For this review, use the dimensioned drawing (mm, ordinates from the lowest corner) and the shaded views. A direction names the side the tool comes from. Round coordinates to 2 decimals unless told otherwise and drop trailing zeros. Loops run counter-clockwise (first coordinate to the right, second up) from the corner with the lowest first, then second, coordinate; pieces in that order, holes last. Notation, with made-up numbers: (46, 50.5) - (100, 50.5) arc R29 ccw to (100, 70.5) - close; hole circle Ø2 at (55, 39). An arc over 180 degrees is marked (long way). Use one line per item in the form item = value. Start each with the question number.
(1) We need section C-C, the plane y = 14. Write out the cut boundary in (x, z).
(2) We need section B-B, the plane z = 21. Write out the cut boundary in (x, y) (1 decimal), then the cut area to 3 significant figures.
(3) We need section A-A, the plane x = 21. Write out the cut boundary in (y, z) (1 decimal), then the cut area to 3 significant figures.
(4) Machinability: for the marked faces 1 and 2, which of the approach directions +Z, -Z, +X, -X, +Y, -Y give a long, thin tool a straight path to every point of the face, cutting with its end or side? Answer none if there is none.
(5) For pin 1 (1.5 mm diameter, centred on x = 39.5, z = 43, fed in from -Y), flat-tipped, find the tip position at first contact; note if it passes through.
(6) Wall thickness on probe 1 along Y at (x, z) = (55, 10); probe 2 along Z at (x, y) = (30, 14.5) (1 decimal); probe 3 along Z at (x, y) = (21.5, 3.5) (1 decimal): over which ranges is each line inside the solid? List them lowest first. Write a range as [from, to].
(7) We need section D-D, the plane x = 12.5. Write out the cut boundary in (y, z) (1 decimal), then the cut area to 3 significant figures.
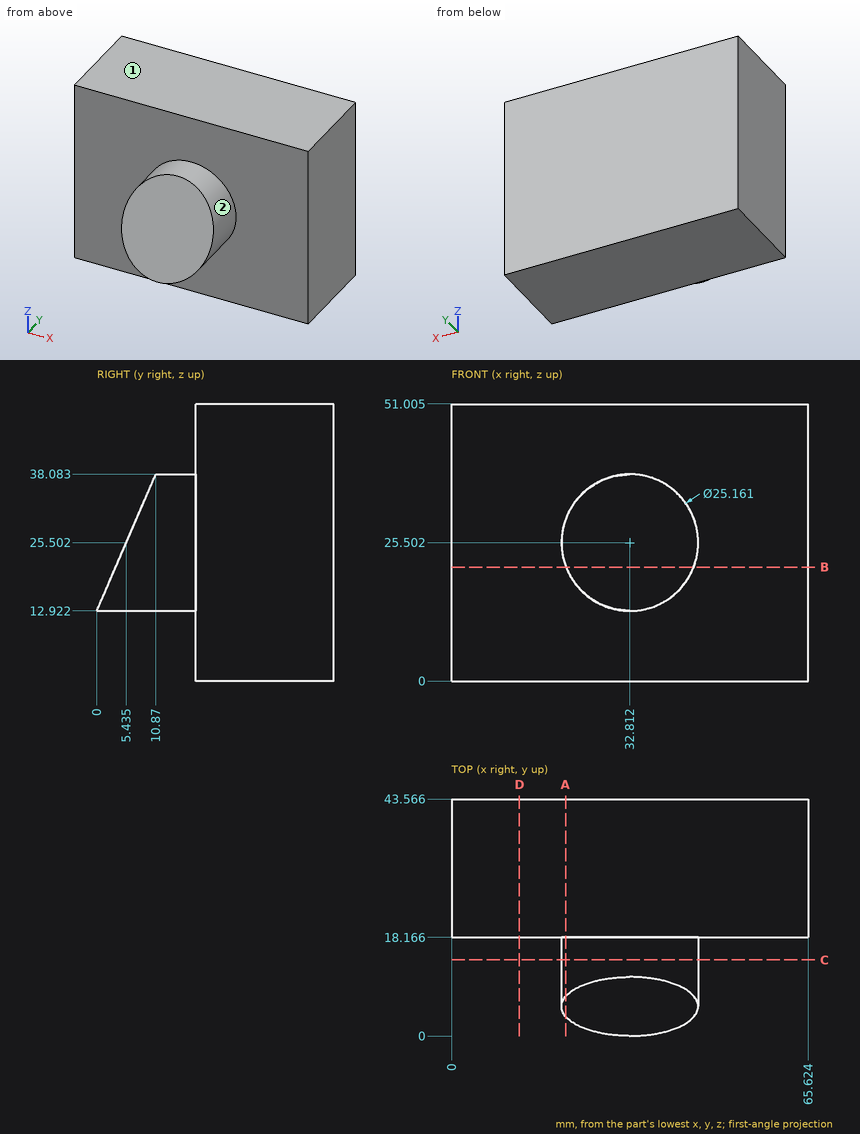
Data:
q1.outline = circle Ø25.16 at (32.81, 25.5)
q2.outline = (0, 18.2) - (21.1, 18.2) - (21.1, 3.5) - (44.6, 3.5) - (44.6, 18.2) - (65.6, 18.2) - (65.6, 43.6) - (0, 43.6) - close
q2.area = 2,010 mm^2
q3.outline = (3.6, 21.2) - (18.2, 21.2) - (18.2, 0) - (43.6, 0) - (43.6, 51) - (18.2, 51) - (18.2, 29.8) - (7.3, 29.8) - close
q3.area = 1,410 mm^2
q4.face_1 = +Z, +X, -X, +Y, -Y
q4.face_2 = -Y
q5.pin_1 = 18.17
q6.probe_1 = [18.17, 43.57]
q6.probe_2 = [13.2, 37.8]
q6.probe_3 = [20, 21]
q7.outline = (18.2, 0) - (43.6, 0) - (43.6, 51) - (18.2, 51) - close
q7.area = 1,300 mm^2
